from build123d import *

# Parameters (mm, degrees)
F0_W         = 113
F0_H         = 75
F1_DEPTH     = 0.6
F2_W         = 113
F2_H         = 15
F3_DEPTH     = 1.8
F4_R         = 7
F5_DEPTH     = 6
F6_R         = 5
F7_DEPTH     = 1.6
F8_R         = 2.5
F9_DEPTH     = 1
F10_W        = 13
F10_H        = 10
F10_W_2      = 9
F10_H_2      = 12
F10_H_3      = 6
F10_W_3      = 7
F11_DEPTH    = 3
F13_W        = 39
F13_H        = 21
F14_DEPTH    = 7
F15_DEPTH    = 4
F18_DEPTH    = 14
F19_W        = 7
F19_H        = 27
F21_W        = 1.8
F21_H        = 21
F23_T1_DEPTH = 23.4311896062
F23_T6_DEPTH = 23.4311896062
F24_W        = 3
F24_H        = 2.8
F25_DEPTH    = 5.6
F26_W        = 6
F26_H        = 3
F27_DEPTH    = 3
F28_W        = 6
F28_H        = 3
F29_DEPTH    = 6
F30_R        = 2
F31_DEPTH    = 4


# Not quite as in the source:
# - a fillet or chamfer that OpenCascade refuses, or shapes differently, is made with other operations: its cross-section is extruded or revolved along the edge and cut away or added


with BuildPart() as f1:
    # F0 (on Top) → F1 (new body)
    with BuildSketch(Plane.XY):
        with Locations((0, 37.5)):
            Rectangle(F0_W, F0_H)
    extrude(amount=F1_DEPTH)

    # F2 (on face) → F3 (join)
    with BuildSketch(Plane.XY.offset(0.6)):
        with Locations((0, 67.5)):
            Rectangle(F2_W, F2_H)
    extrude(amount=F3_DEPTH)

    # F4 (on face) → F5 (join)
    with BuildSketch(Plane.XY.offset(0.6)):
        with Locations((-19.5, 60)):
            Circle(F4_R)
    extrude(amount=F5_DEPTH)

    # F6 (on face) → F7 (join)
    with BuildSketch(Plane.XY.offset(6.6)):
        with Locations((-19.5, 60)):
            Circle(F6_R)
    extrude(amount=F7_DEPTH)

    # F8 (on face) → F9 (join)
    with BuildSketch(Plane.XY.offset(8.2)):
        with Locations((-19.5, 60)):
            Circle(F8_R)
    extrude(amount=F9_DEPTH)

    # F10 (on face) → F11 (join)
    with BuildSketch(Plane.XY.offset(0.6)):
        with Locations((-42, 18)):
            Rectangle(F10_W, F10_H)
        with Locations((-32, 33)):
            Rectangle(F10_W_2, F10_H_2)
        with Locations((25, 39)):
            Rectangle(F10_W, F10_H_3)
        with Locations((40, 39)):
            Rectangle(F10_W_3, F10_H_3)
    extrude(amount=F11_DEPTH)

    # F13 (on face) → F14 (join)
    with BuildSketch(Plane.XY.offset(0.6)):
        with Locations((18, 18.5)):
            Rectangle(F13_W, F13_H)
    extrude(amount=F14_DEPTH)

    # F12 (on face) → F15 (join)
    with BuildSketch(Plane.XY.offset(0.6)):
        Polygon((-12.5, 40), (-20.5, 40), (-20.5, 25), (0.5, 25), (0.5, 36), (-12.5, 36), align=None)
    extrude(amount=F15_DEPTH)

    # F17 (on offset) → F18 (join)
    with BuildSketch(Plane.YZ.offset(15)):
        Polygon((29, 0.6), (44, 0.6), (29, 7.6), align=None)
    extrude(amount=-F18_DEPTH)

    # F19 (on face) → F22 section 0
    with BuildSketch(Plane.XY.offset(0.6)):
        with Locations((-45, 42.5)):
            Rectangle(F19_W, F19_H)
    # F21 (on offset) → F22 section 1
    with BuildSketch(Plane.XY.offset(6.6)):
        with Locations((-46.2, 42.5)):
            Rectangle(F21_W, F21_H)
    loft()

    # F23: fillet of radius 7 on 2 edges, made by hand

    # F23_s2 → F23_t1 (cut)
    with BuildSketch(Plane.YZ.offset(-57.9155948031)):
        with BuildLine():
            ThreePointArc((54.9347524158, 2.7304951685), (52.3538798636, 5.5545556585), (48.6737620788, 6.6))
            Line((48.6737620788, 6.6), (53, 6.6))
            Line((53, 6.6), (54.9347524158, 2.7304951685))
        make_face()
    extrude(amount=F23_T1_DEPTH, mode=Mode.SUBTRACT)


with BuildPart() as f23_tool4:
    # F23_s5 → F23_t6 (new body)
    with BuildSketch(Plane.YZ.offset(-57.9155948031)):
        with BuildLine():
            ThreePointArc((30.0652475842, 2.7304951685), (32.6461201364, 5.5545556585), (36.3262379212, 6.6))
            Line((36.3262379212, 6.6), (32, 6.6))
            Line((32, 6.6), (30.0652475842, 2.7304951685))
        make_face()
    extrude(amount=F23_T6_DEPTH)

    split(bisect_by=Plane.YZ.offset(-36.5), keep=Keep.BOTTOM)


with BuildPart() as f1_1:
    add(f1.part)

    # F23_t3: cut F23_tool4
    add(f23_tool4.part, mode=Mode.SUBTRACT)

    # F24 (on face) → F25 (join)
    with BuildSketch(Plane.XY.offset(2.4)):
        with Locations((-55, 70.6)):
            Rectangle(F24_W, F24_H)
        with Locations((-55, 64.6)):
            Rectangle(F24_W, F24_H)
    extrude(amount=F25_DEPTH)

    # F26 (on face) → F27 (cut)
    with BuildSketch(Plane.XY.offset(2.4)):
        with Locations((53.5, 70.5)):
            Rectangle(F26_W, F26_H)
        with Locations((53.5, 64.5)):
            Rectangle(F26_W, F26_H)
    extrude(amount=-F27_DEPTH, mode=Mode.SUBTRACT)

    # F28 (on face) → F29 (join)
    with BuildSketch(Plane.XY.offset(0.6)):
        with Locations((-53.5, 1.5)):
            Rectangle(F28_W, F28_H)
        with Locations((38.5, 1.5)):
            Rectangle(F28_W, F28_H)
    extrude(amount=F29_DEPTH)

    # F30 (on face) → F31 (cut)
    with BuildSketch(Plane.XZ):
        with Locations((-53.5, 3.6)):
            Circle(F30_R)
        with Locations((38.5, 3.6)):
            Circle(F30_R)
    extrude(amount=-F31_DEPTH, mode=Mode.SUBTRACT)


solid = f1_1.part
Could you check a few things on this model? Use its own coordinates, in mm. A direction names the side the tool comes from. Give positions to 0.01 mm unless a question says otherwise; leave off trailing zeros. Order: outer loops, then holes, each group sorted by start corner. A loop starts at its lowest first (then second) coordinate and runs counter-clockwise, first axis right, second up. Notation, with made-up numbers: (-11.5, 78.25) -> (16.5, 78.25) arc R29 cw to (16.5, 112.25) -> close; hole circle Ø4 at (5, 84). An arc over 180 degrees is marked (long way). Answer in a Markdown table with one row per item. Add a question column.
Item 1: I'm going to push flat-ended pins straight in: P1, Ø1.5, axis at y = 38, z = 2.5, coming from the -X side; P2, Ø0.8, axis at x = -55.5, y = 70.5, coming from the +Z side; P3, Ø1.8, axis at x = 27.5, y = 38.5, coming from the +Z side. Where does each tip first touch, or does it pass through?
Item 2: Imagine slicing it at A-A (x = -11). List the corners of the cut face in (y, z) for me.
Item 3: For faces 4 (the flat face through (-11, 25, 3)), 5 (the flat face through (1, 33, 3)), 6 (the flat face through (-55, 63.2, 5)), 7 (the flat face through (-53.5, 65, 5)), 8 (the flat face through (50.5, 70, 1)), which set-ups out of +Z, -Z, +X, -X, +Y, -Y let a thin tool reach every point of the face, with its end or its side?
Item 4: Imagine slicing it at B-B (x = 11.5). List the corners of the cut face in (y, z) for me, and give its area (4 significant figures).
Item 5: We'd pull the mould along X, two halves only. Please class faces 1 (the flat face through (56.5, 67, 1)), 2 (the flat face through (40, 42, 2)), 3 (the cylindrical face through (-20.151, 64.957, 7.389)): pulls with the +X half, pulls with the -X half, needs draft (parallel to the pull), parting line crosses it, or undercut.
Item 6: Please list where these lines run through material, in increasing order: probe 1 along Y at (x, z) = (24, 1); probe 2 along Z at (x, y) = (38.5, 1.2); probe 3 along X at (y, z) = (9.5, 3.75).
Result:
| question | item | result |
|---|---|---|
| 1 | P1 | x = -48.23 |
| 1 | P2 | z = 8 |
| 1 | P3 | z = 3.6 |
| 2 | outline | (0, 0) -> (75, 0) -> (75, 2.4) -> (60, 2.4) -> (60, 0.6) -> (36, 0.6) -> (36, 4.6) -> (25, 4.6) -> (25, 0.6) -> (0, 0.6) -> close |
| 3 | face 4 | +Z, -X, -Y |
| 3 | face 5 | +Z |
| 3 | face 6 | +Z, -X |
| 3 | face 7 | +Z, +Y |
| 3 | face 8 | +Z, -Z, +X |
| 4 | outline | (0, 0) -> (75, 0) -> (75, 2.4) -> (60, 2.4) -> (60, 0.6) -> (44, 0.6) -> (29, 7.6) -> (8, 7.6) -> (8, 0.6) -> (0, 0.6) -> close |
| 4 | area | 271.5 mm2 |
| 5 | face 1 | pulls with the +X half |
| 5 | face 2 | needs draft |
| 5 | face 3 | undercut |
| 6 | probe 1 | 8 to 29, 36 to 42, 60 to 75 |
| 6 | probe 2 | 0 to 1.6, 5.6 to 6.6 |
| 6 | probe 3 | -1.5 to 37.5 |
